from build123d import *

# Parameters (mm, degrees)
BOX_W        = 120
BOX_H        = 40
BOX_DEPTH    = 10
FILLET_R     = 7
BOX002_W     = 130
BOX002_H     = 50
BOX002_DEPTH = 2
FILLET002_R  = 12
BOX001_W     = 126
BOX001_H     = 46
BOX001_DEPTH = 10
FILLET001_R  = 10
FILLET003_R  = 1.5
FILLET004_R  = 1


with BuildPart() as fillet_body:
    # Box → Box (new body)
    with BuildSketch(Plane.XY):
        with Locations((60, 20)):
            Rectangle(BOX_W, BOX_H)
    extrude(amount=BOX_DEPTH)

    # Fillet
    fillet_edges = [fillet_body.edges().sort_by_distance(p)[0] for p in [
        (0, 0, 5),
        (0, 40, 5),
        (120, 0, 5),
        (120, 40, 5),
    ]]
    fillet(fillet_edges, radius=FILLET_R)


with BuildPart() as fillet_body_1:
    # Fillet placement: moved
    add(fillet_body.part.moved(Location((5, 5, 0))))


with BuildPart() as fillet002:
    # Box002 → Box002 (new body)
    with BuildSketch(Plane.XY):
        with Locations((65, 25)):
            Rectangle(BOX002_W, BOX002_H)
    extrude(amount=BOX002_DEPTH)

    # Fillet002
    fillet002_edges = [fillet002.edges().sort_by_distance(p)[0] for p in [
        (0, 0, 1),
        (0, 50, 1),
        (130, 0, 1),
        (130, 50, 1),
    ]]
    fillet(fillet002_edges, radius=FILLET002_R)


with BuildPart() as fillet004:
    # Box001 → Box001 (new body)
    with BuildSketch(Plane.XY):
        with Locations((63, 23)):
            Rectangle(BOX001_W, BOX001_H)
    extrude(amount=BOX001_DEPTH)

    # Fillet001
    fillet001_edges = [fillet004.edges().sort_by_distance(p)[0] for p in [
        (0, 0, 5),
        (0, 46, 5),
        (126, 0, 5),
        (126, 46, 5),
    ]]
    fillet(fillet001_edges, radius=FILLET001_R)


with BuildPart() as fillet004_1:
    # Fillet001 placement: moved
    add(fillet004.part.moved(Location((2, 2, 0))))

    # Fusion: union Fillet002
    add(fillet002.part)

    # Cut: cut Fillet body
    add(fillet_body_1.part, mode=Mode.SUBTRACT)

    # Fillet003
    fillet003_edges = [fillet004_1.edges().sort_by_distance(p)[0] for p in [
        (7.050253, 7.050253, 0),
        (65, 5, 0),
        (122.949747, 7.050253, 0),
        (125, 25, 0),
        (122.949747, 42.949747, 0),
        (65, 45, 0),
        (7.050253, 42.949747, 0),
        (5, 25, 0),
    ]]
    fillet(fillet003_edges, radius=FILLET003_R)

    # Fillet004
    fillet004_edges = [fillet004_1.edges().sort_by_distance(p)[0] for p in [
        (0, 25, 0),
        (3.514719, 3.514719, 0),
        (3.514719, 46.485281, 0),
        (65, 0, 0),
        (65, 50, 0),
        (126.485281, 3.514719, 0),
        (126.485281, 46.485281, 0),
        (130, 25, 0),
    ]]
    fillet(fillet004_edges, radius=FILLET004_R)


solid = fillet004_1.part
Verification items for the finished model (mm, model axes). A direction names the side the tool comes from. Coordinates: 2 decimals unless noted, no trailing zeros. Order: outer loops, then holes, each group sorted by start corner. A loop starts at its lowest first (then second) coordinate and runs counter-clockwise, first axis right, second up. Notation, with made-up numbers: (3, 69) -> (37, 69) arc R21 ccw to (37, 108) -> close; hole circle Ø10 at (62.25, 1). An arc over 180 degrees is marked (long way). Put each result on its own line as item: value. Start each with the question number.
1. Mould release check, pull along X, two halves, no side actions. Record for faces 4 (the cylindrical face through (4.85, 5.01, 6.06)), 5 (the flat face through (64, 45, 6)), 6 (the flat face through (65, 1, 2)): released by +X, released by -X, zero draft, split by the parting line, or undercut.
2. Material ranges on L1, parallel to X at y = 15.5, z = 8; L2, parallel to Y at x = 79.5, z = 6.75; L3, parallel to Y at x = 46, z = 1.25, recorded low to high. Write a range as [from, to].
3. Cross-section at B-B, the plane y = 14. Record the boundary of the cut face in (x, z), then the cut area to 3 significant figures.
4. Cross-section at A-A, the plane x = 104. Record the boundary of the cut face in (y, z), then the cut area to 3 significant figures.
5. Go/stop test with flat-tipped pins: pin 1 Ø25 at (x, y) = (77.5, 25.5) entering from +Z; pin 2 Ø5 at (y, z) = (38.5, 3.5) entering from +X; pin 3 Ø4 at (x, z) = (45.5, 7.5) entering from +Y; pin 4 Ø4 at (y, z) = (27.5, 6.5) entering from -X. Record where each tip stops, or that it passes through.
6. Cross-section at C-C, the plane z = 5. Record the boundary of the cut face in (x, y), then the cut area to 3 significant figures.
7. Access from +Z, -Z, +X, -X, +Y, -Y to the whole of each face (thin tool, end or side, straight path). Record for faces 1 (the flat face through (2, 25, 6)), 2 (the flat face through (64, 2, 6)), 3 (the flat face through (128, 25, 6)).
Computed:
1. face 4: released by -X
1. face 5: undercut
1. face 6: zero draft
2. L1: [2, 5], [125, 128]
2. L2: [2, 5], [45, 48]
2. L3: [0, 4.98], [45.02, 50]
3. outline: (0, 1) arc R1 ccw to (1, 0) -> (3.5, 0) arc R1.5 ccw to (5, 1.5) -> (5, 10) -> (2, 10) -> (2, 2) -> (0, 2) -> close; (125, 1.5) arc R1.5 ccw to (126.5, 0) -> (129, 0) arc R1 ccw to (130, 1) -> (130, 2) -> (128, 2) -> (128, 10) -> (125, 10) -> close
3. area: 66.6 mm2
4. outline: (0, 1) arc R1 ccw to (1, 0) -> (3.5, 0) arc R1.5 ccw to (5, 1.5) -> (5, 10) -> (2, 10) -> (2, 2) -> (0, 2) -> close; (45, 1.5) arc R1.5 ccw to (46.5, 0) -> (49, 0) arc R1 ccw to (50, 1) -> (50, 2) -> (48, 2) -> (48, 10) -> (45, 10) -> close
4. area: 66.6 mm2
5. pin 1: through
5. pin 2: x = 130
5. pin 3: y = 48
5. pin 4: x = 2
6. outline: (2, 12) arc R10 ccw to (12, 2) -> (118, 2) arc R10 ccw to (128, 12) -> (128, 38) arc R10 ccw to (118, 48) -> (12, 48) arc R10 ccw to (2, 38) -> close; hole (5, 12) arc R7 ccw to (12, 5) -> (118, 5) arc R7 ccw to (125, 12) -> (125, 38) arc R7 ccw to (118, 45) -> (12, 45) arc R7 ccw to (5, 38) -> close
6. area: 952 mm2
7. face 1: +Z, -X, +Y, -Y
7. face 2: +Z, +X, -X, -Y
7. face 3: +Z, +X, +Y, -Y
